from build123d import *

# Parameters (mm, degrees)
SKETCH1_R           = 25
BOSS_EXTRUDE1_DEPTH = 5
SKETCH2_R           = 10
SKETCH2_R_2         = 6
BOSS_EXTRUDE2_DEPTH = 50
FILLET1_R           = 1


with BuildPart() as part:
    # Sketch1 → Boss-Extrude1 (new body)
    with BuildSketch(Plane(origin=(0, 0, 0), x_dir=(1, 0, 0), z_dir=(0, 1, 0))):
        with Locations(Location((0, 0, 0), (0, 0, 270))):
            Circle(SKETCH1_R)
    extrude(amount=BOSS_EXTRUDE1_DEPTH)

    # Sketch2 → Boss-Extrude2 (add)
    with BuildSketch(Plane(origin=(0, 5, 0), x_dir=(1, 0, 0), z_dir=(0, 1, 0))):
        with Locations(Location((0, 0, 0), (0, 0, 270))):
            Circle(SKETCH2_R)
        with Locations(Location((0, 0, 0), (0, 0, 270))):
            Circle(SKETCH2_R_2, mode=Mode.SUBTRACT)
    extrude(amount=BOSS_EXTRUDE2_DEPTH)

    # Fillet1
    fillet1_edges = [part.edges().sort_by_distance(p)[0] for p in [
        (0, 5, -25),
        (0, 55, -10),
        (0, 5, -10),
    ]]
    fillet(fillet1_edges, radius=FILLET1_R)


solid = part.part
The listing builds one solid part. Answer for the finished solid, in the listing's coordinates (mm). A direction names the side the tool comes from. Round coordinates to 2 decimals unless told otherwise and drop trailing zeros. Write each loop counter-clockwise with the first axis right and the second up, starting at its lowest first coordinate (ties: lowest second). Pieces come first, ordered by that corner, then holes. Notation, with made-up numbers: (21.5, 24) - (75.5, 24) arc R12 ccw to (75.5, 39) - close; hole circle Ø7 at (77, -18). An arc over 180 degrees is marked (long way). Use a Markdown table: item, result. Add a question column.
1. The part is cut by section C-C (y = 7). Write down the section's boundary in (x, z).
2. Consider line 1 (X direction, y = 18.5, z = 0); line 2 (Y direction, x = -3.5, z = 22); line 3 (Z direction, x = 3, y = 48). Determine where each line is inside the solid, lowest interval first.
3. The part is cut by section A-A (x = 0). Write down the section's boundary in (y, z).
4. Flat-ended cylindrical pins translate along their axes: P1, Ø5, axis at x = -12.5, z = -14, coming from the -Y side; P2, Ø1.5, axis at x = -12.5, z = -6, coming from the +Y side; P3, Ø2, axis at y = 35.5, z = 0.5, coming from the -X side. Find the tip coordinate at first contact, or state that the pin passes through.
5. A tool of negligible diameter and unlimited length cuts with its end or side. For faces 4 (the face through (0, 5, 0)), 5 (the face through (0, 0, 0)), from which of +Z, -Z, +X, -X, +Y, -Y can it reach the whole face along a straight path? Write none if from no direction.
6. For a pull along X with two mould halves and no side action, classify faces 1 (the face through (1.802, 29.65, 5.723)), 2 (the face through (-9.76, 29.66, -2.17)), 3 (the face through (-5, 5, 10)) as +X half, -X half, draft (parallel to the pull), parting line (faces both ways), or undercut.
7. The part is cut by section B-B (z = 0). Write down the section's boundary in (x, y), and give its area (3 significant figures).
Reported:
| question | item | result |
|---|---|---|
| 1 | outline | circle Ø20 at (0, 0); hole circle Ø12 at (0, 0) |
| 2 | line 1 | -10 to -6, 6 to 10 |
| 2 | line 2 | 0 to 5 |
| 2 | line 3 | -9.54 to -5.2, 5.2 to 9.54 |
| 3 | outline | (0, -25) - (4, -25) arc R1 ccw to (5, -24) - (5, -11) arc R1 cw to (6, -10) - (54, -10) arc R1 ccw to (55, -9) - (55, -6) - (5, -6) - (5, 6) - (55, 6) - (55, 9) arc R1 ccw to (54, 10) - (6, 10) arc R1 cw to (5, 11) - (5, 24) arc R1 ccw to (4, 25) - (0, 25) - close |
| 4 | P1 | y = 0 |
| 4 | P2 | y = 5 |
| 4 | P3 | x = -10 |
| 5 | face 4 | +Y |
| 5 | face 5 | +Z, -Z, +X, -X, -Y |
| 6 | face 1 | undercut |
| 6 | face 2 | parting line |
| 6 | face 3 | draft |
| 7 | outline | (-25, 0) - (25, 0) - (25, 4) arc R1 ccw to (24, 5) - (11, 5) arc R1 cw to (10, 6) - (10, 54) arc R1 ccw to (9, 55) - (6, 55) - (6, 5) - (-6, 5) - (-6, 55) - (-9, 55) arc R1 ccw to (-10, 54) - (-10, 6) arc R1 cw to (-11, 5) - (-24, 5) arc R1 ccw to (-25, 4) - close |
| 7 | area | 650 mm^2 |
